```python
from build123d import *

# Parameters (mm, degrees)
ESQUISSE1_R                  = 5.5
BASE_EXTRUSION_DEPTH         = 18
ESQUISSE2_R                  = 3
BOSS_EXTRU_1_DEPTH           = 1.8
COQUE1_T                     = -0.5
ESQUISSE3_R                  = 1.25
ENL_V_MAT_EXTRU_1_DEPTH      = 22.272987566
ESQUISSE4_R                  = 1
ESQUISSE4_R_2                = 1.15
ENL_V_MAT_EXTRU_2_DEPTH      = 1
ENL_V_MAT_EXTRU_3_REACH      = 21.609
ESQUISSE5_R                  = 0.5
R_P_TITION_CIRCULAIRE1_COUNT = 3
R_P_TITION_CIRCULAIRE1_ANGLE = 180


with BuildPart() as part:
    # Esquisse1 → Base-Extrusion (new body)
    with BuildSketch(Plane(origin=(0, 0, 0), x_dir=(1, 0, 0), z_dir=(0, 1, 0))):
        with Locations(Location((0, 0, 0), (0, 0, 270))):
            Circle(ESQUISSE1_R)
    extrude(amount=-BASE_EXTRUSION_DEPTH)

    # Esquisse2 → Boss.-Extru.1 (add)
    with BuildSketch(Plane.XZ.offset(18)):
        with Locations(Location((0, 0, 0), (0, 0, 90))):
            Circle(ESQUISSE2_R)
    extrude(amount=BOSS_EXTRU_1_DEPTH)

    # Coque1
    coque1_openings = [part.faces().sort_by_distance(p)[0] for p in [
        (0, 0, 0),
    ]]
    offset(amount=COQUE1_T, openings=coque1_openings, kind=Kind.INTERSECTION)

    # Esquisse3 → Enlèv. mat.-Extru.1 (cut, through all)
    with BuildSketch(Plane.XZ.offset(19.8)):
        with Locations(Location((0, 0, 0), (0, 0, 270))):
            Circle(ESQUISSE3_R)
    extrude(amount=-ENL_V_MAT_EXTRU_1_DEPTH, mode=Mode.SUBTRACT)

    # Esquisse4 → Enlèv. mat.-Extru.2 (cut)
    with BuildSketch(Plane.XZ):
        with Locations((5.5, 0)):
            Circle(ESQUISSE4_R)
        with Locations((0, -5.75)):
            Circle(ESQUISSE4_R_2)
        with Locations((0, 5.75)):
            Circle(ESQUISSE4_R_2)
    extrude(amount=ENL_V_MAT_EXTRU_2_DEPTH, mode=Mode.SUBTRACT)

    # Esquisse5 → Enlèv. mat.-Extru.3 (cut, up to next)
    with BuildSketch(Plane.XZ.offset(18), mode=Mode.PRIVATE) as enl_v_mat_extru_3_sk1:
        with Locations(Location((0, 4.17675231, 0), (0, 0, 270))):
            Circle(ESQUISSE5_R)
    enl_v_mat_extru_3_tool1 = extrude(enl_v_mat_extru_3_sk1.sketch, amount=-ENL_V_MAT_EXTRU_3_REACH, mode=Mode.PRIVATE) & part.part
    enl_v_mat_extru_3 = enl_v_mat_extru_3_tool1.solids().sort_by_distance((0, -18, 4.176752))[0]
    add(enl_v_mat_extru_3, mode=Mode.SUBTRACT)

    # Répétition circulaire1: Enlèv. mat.-Extru.3 ×3 about axis
    r_p_tition_circulaire1_axis = Axis((0, 0, 0), (0, 1, 0))
    for i in range(1, R_P_TITION_CIRCULAIRE1_COUNT):
        add(enl_v_mat_extru_3.rotate(r_p_tition_circulaire1_axis, i * R_P_TITION_CIRCULAIRE1_ANGLE / (R_P_TITION_CIRCULAIRE1_COUNT - 1)), mode=Mode.SUBTRACT)


solid = part.part
```
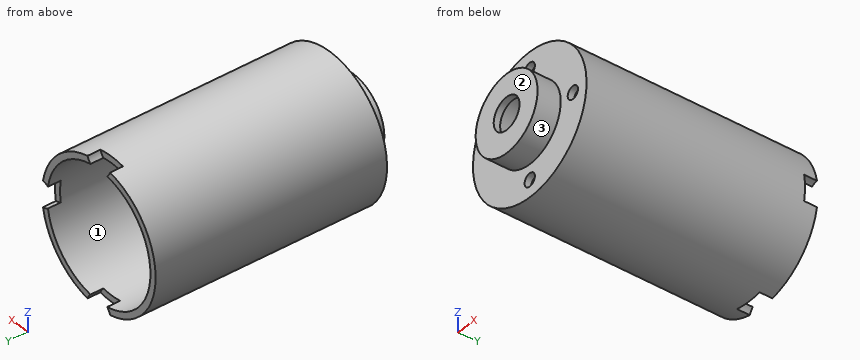
Design review of the part built by this model. Coordinates are the model's own, in mm. Face numbers are marked on the shaded views. A direction names the side the tool comes from. Round coordinates to 2 decimals unless told otherwise and drop trailing zeros. Write each loop counter-clockwise with the first axis right and the second up, starting at its lowest first coordinate (ties: lowest second). Pieces come first, ordered by that corner, then holes. Notation, with made-up numbers: (70, -33.5) -> (95, -33.5) arc R12 ccw to (95, -16.5) -> close; hole circle Ø6 at (-31, 59.5). An arc over 180 degrees is marked (long way). Write item = value, one per line. Start each with the question number.
1) Take a section at A-A, the plane z = 0. State the section outline as (x, y) points.
2) Take a section at C-C, the plane y = -13.25. State the section outline as (x, z) points, plus the area to 3 significant figures.
3) Clearance check with flat-ended pins moving along their axes: pin 1 (5.5 mm diameter, centred on x = -0.5, z = 1, fed in from +Y); pin 2 (3 mm diameter, centred on x = -4, y = -16, fed in from -Z); pin 3 (0.6 mm diameter, centred on x = 5, z = 0, fed in from +Y). State where each tip first meets the part, or that it passes through.
4) Take a section at D-D, the plane z = -4. State the section outline as (x, y) points, plus the area to 3 significant figures.
5) Tool access review of the marked faces 1, 2 and 3: name each direction out of +Z, -Z, +X, -X, +Y, -Y from which nothing blocks a thin tool from reaching the whole face with its end or side.
6) Wall thickness on probe 1 along X at (y, z) = (-9, 0); probe 2 along X at (y, z) = (-18.4, 0); probe 3 along Y at (x, z) = (2, -3.5): over which ranges is each line inside the solid? List them lowest first. Write a range as from..to.
7) Take a section at B-B, the plane x = 0. State the section outline as (y, z) points.
Results list:
q1.outline = (-5.5, -18) -> (-3, -18) -> (-3, -19.8) -> (-1.25, -19.8) -> (-1.25, -19.3) -> (-2.5, -19.3) -> (-2.5, -17.5) -> (-5, -17.5) -> (-5, 0) -> (-5.5, 0) -> close; (1.25, -19.8) -> (3, -19.8) -> (3, -18) -> (3.68, -18) -> (3.68, -17.5) -> (2.5, -17.5) -> (2.5, -19.3) -> (1.25, -19.3) -> close; (4.68, -18) -> (5.5, -18) -> (5.5, -1) -> (5, -1) -> (5, -17.5) -> (4.68, -17.5) -> close
q2.outline = circle Ø11 at (0, 0); hole circle Ø10 at (0, 0)
q2.area = 16.5 mm²
q3.pin_1 = -17.5
q3.pin_2 = -4.9
q3.pin_3 = -1
q4.outline = (-3.77, -18) -> (-0.47, -18) -> (-0.47, -17.5) -> (-3, -17.5) -> (-3, 0) -> (-3.77, 0) -> close; (0.47, -18) -> (3.77, -18) -> (3.77, 0) -> (3, 0) -> (3, -17.5) -> (0.47, -17.5) -> close
q4.area = 30.4 mm²
q5.face_1 = +Y
q5.face_2 = +Z, -Z, +X, -X, -Y
q5.face_3 = -Y
q6.probe_1 = -5.5..-5, 5..5.5
q6.probe_2 = -3..-2.5, 2.5..3
q6.probe_3 = -18..-17.5
q7.outline = (-19.8, -3) -> (-18, -3) -> (-18, -3.68) -> (-17.5, -3.68) -> (-17.5, -2.5) -> (-19.3, -2.5) -> (-19.3, -1.25) -> (-19.8, -1.25) -> close; (-19.8, 1.25) -> (-19.3, 1.25) -> (-19.3, 2.5) -> (-17.5, 2.5) -> (-17.5, 3.68) -> (-18, 3.68) -> (-18, 3) -> (-19.8, 3) -> close; (-18, -5.5) -> (-1, -5.5) -> (-1, -5) -> (-17.5, -5) -> (-17.5, -4.68) -> (-18, -4.68) -> close; (-18, 4.68) -> (-17.5, 4.68) -> (-17.5, 5) -> (-1, 5) -> (-1, 5.5) -> (-18, 5.5) -> close
